```python
from build123d import *

# Parameters (mm, degrees)
ESQUISSE1_R             = 4.3
ESQUISSE1_R_2           = 2.6
ESQUISSE1_R_3           = 2
BOSS_EXTRU_1_DEPTH      = 1.2
ESQUISSE2_R             = 2.6
ESQUISSE2_R_2           = 2
BOSS_EXTRU_3_DEPTH      = 3.2
ESQUISSE3_R             = 4.3
ESQUISSE3_R_2           = 2
BOSS_EXTRU_4_DEPTH      = 0.8
ESQUISSE4_R             = 4.8
ESQUISSE4_R_2           = 2
BOSS_EXTRU_5_DEPTH      = 2
ESQUISSE6_R             = 3
ENL_V_MAT_EXTRU_1_DEPTH = 3


with BuildPart() as part:
    # Esquisse1 → Boss.-Extru.1 (new body)
    # profile 1 of 2: a face of its own
    with BuildSketch(Plane.XY):
        Circle(ESQUISSE1_R)
        Circle(ESQUISSE1_R_2, mode=Mode.SUBTRACT)
    # profile 2 of 2: a face of its own
    with BuildSketch(Plane.XY):
        Circle(ESQUISSE1_R_2)
        Circle(ESQUISSE1_R_3, mode=Mode.SUBTRACT)
    extrude(amount=BOSS_EXTRU_1_DEPTH)

    # Esquisse2 → Boss.-Extru.3 (add)
    with BuildSketch(Plane.XY.offset(1.2)):
        Circle(ESQUISSE2_R)
        Circle(ESQUISSE2_R_2, mode=Mode.SUBTRACT)
    extrude(amount=BOSS_EXTRU_3_DEPTH)

    # Esquisse3 → Boss.-Extru.4 (add)
    with BuildSketch(Plane.XY.offset(4.4)):
        Circle(ESQUISSE3_R)
        Circle(ESQUISSE3_R_2, mode=Mode.SUBTRACT)
    extrude(amount=BOSS_EXTRU_4_DEPTH)

    # Esquisse4 → Boss.-Extru.5 (add)
    with BuildSketch(Plane.XY.offset(5.2)):
        Circle(ESQUISSE4_R)
        Circle(ESQUISSE4_R_2, mode=Mode.SUBTRACT)
    extrude(amount=BOSS_EXTRU_5_DEPTH)

    # Esquisse5 → Révolution2 (revolve)
    with BuildSketch(Plane(origin=(0, 0, 0), x_dir=(1, 0, 0), z_dir=(0, 1, 0)), mode=Mode.PRIVATE) as r_volution2_sk:
        Polygon((-4.3, 0), (-3.599996072, 3), (0, 2.994682018), (0, 0), align=None)
    revolve(r_volution2_sk.sketch.rotate(Axis((0, 0, 7.316321581), (0, 0, -1)), 180), axis=Axis((0, 0, 7.316321581), (0, 0, -1)))

    # Esquisse6 → Enlèv. mat.-Extru.1 (cut)
    with BuildSketch(Plane(origin=(0, 0, 0), x_dir=(-1, 0, 0), z_dir=(0, 0, -1))):
        Circle(ESQUISSE6_R)
    extrude(amount=ENL_V_MAT_EXTRU_1_DEPTH, mode=Mode.SUBTRACT)


solid = part.part
```
Could you check a few things on this model? Use its own coordinates, in mm. A direction names the side the tool comes from. Round coordinates to 2 decimals unless told otherwise and drop trailing zeros. Loops run counter-clockwise (first coordinate to the right, second up) from the corner with the lowest first, then second, coordinate; pieces in that order, holes last. Notation, with made-up numbers: M 3.5,24 L 44.5,24 A19 cw 44.5,32 Z; hole C 41,-25 d5. An arc over 180 degrees is marked long. Answer as CSV lines item,"result".
1) Imagine slicing it at A-A on y = 0. List the corners of the cut face in (x, z) for me, and give its area (3 significant figures).
From the geometry:
outline,"M -4.8,5.2 L -4.3,5.2 L -4.3,4.4 L -2.6,4.4 L -2.6,1.2 L -4.3,1.2 L -4.3,0 L -3.6,-3 L -3,-3 L -3,0 L -2,0 L -2,7.2 L -4.8,7.2 Z; M 2,0 L 3,0 L 3,-3 L 3.6,-3 L 4.3,0 L 4.3,1.2 L 2.6,1.2 L 2.6,4.4 L 4.3,4.4 L 4.3,5.2 L 4.8,5.2 L 4.8,7.2 L 2,7.2 Z"
area,"29.9 mm^2"
2) If I drill on probe 1 along Z at (x, y) = (1, 2.75); probe 2 along Y at (x, z) = (0, 4.75); probe 3 along Y at (x, z) = (0, 4.25), over which ranges is the centre line in solid material (lowest first)?
From the geometry:
probe 1,"0 to 1.2, 4.4 to 7.2"
probe 2,"-4.3 to -2, 2 to 4.3"
probe 3,"-2.6 to -2, 2 to 2.6"
3) For pin 1 Ø3 at (x, y) = (-0.5, 0.5) entering from -Z; pin 2 Ø1 at (y, z) = (-4, 0) entering from +X; pin 3 Ø4 at (y, z) = (2.5, 4.5) entering from -X, each with a flat end and sliding along its axis, tell me the tip position at first contact or that it passes through.
From the geometry:
pin 1,"z = 0"
pin 2,"x = 2.5"
pin 3,"x = -4.76"
4) Imagine slicing it at C-C on z = 4. List the corners of the cut face in (x, y) for me.
From the geometry:
outline,"C 0,0 d5.2; hole C 0,0 d4"
5) Which directions (+Z, -Z, +X, -X, +Y, -Y) give clear straight access to the entire face, cutting with the end or side of a thin tool? Please do faces 1 (the cylindrical face through (0, -2, 4)), 2 (the cylindrical face through (-4.296, 0.189, 4.794)), 3 (the cylindrical face through (-0.338, 2.578, 2.778)).
From the geometry:
face 1,"+Z, -Z"
face 2,"-Z"
face 3,"none"
6) We'd pull the mould along X, two halves only. Please class faces 4 (the cylindrical face through (3, 0, -1)), 5 (the cylindrical face through (-4.296, 0.189, 0.592)), 6 (the flat face through (-4, 2, 5.2)): released by +X, released by -X, zero draft, split by the parting line, or undercut.
From the geometry:
face 4,"undercut"
face 5,"split by the parting line"
face 6,"zero draft"
7) Imagine slicing it at D-D on z = 6.5. List the corners of the cut face in (x, y) for me, and give its area (3 significant figures).
From the geometry:
outline,"C 0,0 d9.6; hole C 0,0 d4"
area,"59.8 mm^2"
